from build123d import *

# Parameters (mm, degrees)
SKETCH_1_W          = 2.5
SKETCH_1_H          = 103
SKETCH_1_W_2        = 2
SKETCH_1_H_2        = 95
EXTRUDE_1_DEPTH     = 99.5
CUT_EXTRUDE_2_DEPTH = 4.5
CUT_EXTRUDE_3_DEPTH = 58.5
CUT_EXTRUDE_4_DEPTH = 4.5
SKETCH_6_W          = 1.6
SKETCH_6_H          = 17
CUT_EXTRUDE_5_DEPTH = 10
EXTRUDE_START       = -62
SKETCH_7_W          = 1
SKETCH_7_H          = 1
EXTRUDE_2_DEPTH     = 119.954657
EXTRUDE_START_2     = -58
SKETCH_8_W          = 0.5
SKETCH_8_H          = 0.5
EXTRUDE_3_DEPTH     = 119.954657


with BuildPart() as part:
    # 스케치1 → 보스-돌출1 (new body)
    with BuildSketch(Plane(origin=(0, 0, 0), x_dir=(1, 0, 0), z_dir=(0, 1, 0))):
        with Locations((1.25, -51.5)):
            Rectangle(SKETCH_1_W, SKETCH_1_H)
        with Locations((3.5, -51.5)):
            Rectangle(SKETCH_1_W_2, SKETCH_1_H_2)
    extrude(amount=EXTRUDE_1_DEPTH)

    # 스케치2 → 컷-돌출2 (cut)
    with BuildSketch(Plane(origin=(4.5, 0, 0), x_dir=(0, 0, -1), z_dir=(1, 0, 0))):
        with BuildLine():
            Line((-62, 10), (-62, 0))
            Line((-62, 0), (-41, 0))
            Line((-41, 0), (-41, 10))
            ThreePointArc((-41, 10), (-51.5, 20.5), (-62, 10))
        make_face()
    extrude(amount=-CUT_EXTRUDE_2_DEPTH, mode=Mode.SUBTRACT)

    # 스케치3 → 컷-돌출3 (cut)
    with BuildSketch(Plane(origin=(0, 99.5, 0), x_dir=(1, 0, 0), z_dir=(0, 1, 0))):
        Polygon((2.5, -4), (2.5, 0), (0, 0), (0, -103), (2.5, -103), (2.5, -99), (4.5, -99), (4.5, -4), align=None)
    extrude(amount=-CUT_EXTRUDE_3_DEPTH, mode=Mode.SUBTRACT)

    # 스케치4 → 컷-돌출4 (cut)
    with BuildSketch(Plane(origin=(0, 41, 0), x_dir=(1, 0, 0), z_dir=(0, 1, 0))):
        Polygon((4.5, -4), (2.5, -4), (2.5, 0), (0, 0), (0, -103), (2.5, -103), (2.5, -99), (4.5, -99), align=None)
    extrude(amount=-CUT_EXTRUDE_4_DEPTH, mode=Mode.SUBTRACT)

    # 스케치6 → 컷-돌출5 (cut)
    with BuildSketch(Plane.XZ):
        with Locations((0.8, 74)):
            Rectangle(SKETCH_6_W, SKETCH_6_H)
    extrude(amount=-CUT_EXTRUDE_5_DEPTH, mode=Mode.SUBTRACT)

    # 스케치7 → 보스-돌출2 (add)
    with BuildSketch(Plane(origin=(0, 0, 0), x_dir=(-1, 0, 0), z_dir=(0, 0, -1)).offset(EXTRUDE_START)):
        with Locations((-1.25, 1.524584525)):
            Rectangle(SKETCH_7_W, SKETCH_7_H)
        with Locations((-1.25, 11.524584525)):
            Rectangle(SKETCH_7_W, SKETCH_7_H)
        with Locations((-1.25, 21.524584525)):
            Rectangle(SKETCH_7_W, SKETCH_7_H)
        with Locations((-1.25, 31.524584525)):
            Rectangle(SKETCH_7_W, SKETCH_7_H)
    extrude(amount=EXTRUDE_2_DEPTH)

    # 스케치8 → 보스-돌출3 (add)
    with BuildSketch(Plane(origin=(0, 0, 4), x_dir=(-1, 0, 0), z_dir=(0, 0, -1)).offset(EXTRUDE_START_2)):
        with Locations((-3.5, 3.368615417)):
            Rectangle(SKETCH_8_W, SKETCH_8_H)
        with Locations((-3.5, 13.368615417)):
            Rectangle(SKETCH_8_W, SKETCH_8_H)
        with Locations((-3.5, 23.368615417)):
            Rectangle(SKETCH_8_W, SKETCH_8_H)
        with Locations((-3.5, 33.368615417)):
            Rectangle(SKETCH_8_W, SKETCH_8_H)
    extrude(amount=EXTRUDE_3_DEPTH)


solid = part.part
Geometry: final body of the model. Coordinates: model frame, mm. A direction names the side the tool comes from. Give positions to 0.01 mm unless a question says otherwise; leave off trailing zeros. Write each loop counter-clockwise with the first axis right and the second up, starting at its lowest first coordinate (ties: lowest second). Pieces come first, ordered by that corner, then holes. Notation, with made-up numbers: M -21,49 L 14,49 A22 cw 14,86 Z; hole C -35,61 d7. An arc over 180 degrees is marked long. Answer in a Markdown table with one row per item. Add a question column.
(1) First-contact query: pin 1 (1.1 mm diameter, centred on y = 21.5, z = -18, fed in from +X); pin 2 (0.5 mm diameter, centred on x = 1, z = -30.5, fed in from +Y); pin 3 (0.5 mm diameter, centred on x = 0.5, z = 70, fed in from -Y); pin 4 (3 mm diameter, centred on y = 17, z = -21, fed in from -X). Flat tips, straight axial feed; report the tip coordinate or a pass-through.
(2) Ray query, line 1 (Y direction, x = 3.65, z = -18); line 2 (Y direction, x = 1.4, z = -36); line 3 (Z direction, x = 1.1, y = 10.5). Return the intervals inside material, ascending.
(3) Section A-A on z = 51.5. Return loops of the section in (x, y).
(4) Section C-C on y = 25.5. Return loops of the section in (x, z), and give its area (4 significant figures).
(5) Mould query, pull axis Z, two halves, no side actions, for faces 4 (the flat face through (1, 18, 103)), 5 (the flat face through (2, 0, 82)), 6 (the cylindrical face through (2.3, 20.5, 51.3)). Classes: +Z half, -Z half, draft (parallel to the pull), parting line (faces both ways), or undercut.
(6) Section B-B on z = -22. State how many separate pieces and enclosed holes the cut face has, and give its area (3 significant figures).
(7) Reachability of faces 1 (the flat face through (1.6, 5, 74)), 2 (the flat face through (2.5, 18, 101)), 3 (the flat face through (2, 0, 20)) from +Z, -Z, +X, -X, +Y, -Y: full face, straight path, thin tool, end or side. Return the list, or none.
Result set:
| question | item | result |
|---|---|---|
| 1 | pin 1 | stops at x = 1.75 |
| 1 | pin 2 | stops at y = 32.02 |
| 1 | pin 3 | stops at y = 10 |
| 1 | pin 4 | passes through |
| 2 | line 1 | y = 3.12 to 3.62, 13.12 to 13.62, 23.12 to 23.62, 33.12 to 33.62 |
| 2 | line 2 | y = 1.02 to 2.02, 11.02 to 12.02, 21.02 to 22.02, 31.02 to 32.02 |
| 2 | line 3 | z = 0 to 41.01, 61.99 to 103 |
| 3 | outline | M 0,20.5 L 4.5,20.5 L 4.5,36.5 L 0,36.5 Z; M 0.75,1.02 L 1.75,1.02 L 1.75,2.02 L 0.75,2.02 Z; M 0.75,11.02 L 1.75,11.02 L 1.75,12.02 L 0.75,12.02 Z; M 3.25,3.12 L 3.75,3.12 L 3.75,3.62 L 3.25,3.62 Z; M 3.25,13.12 L 3.75,13.12 L 3.75,13.62 L 3.25,13.62 Z |
| 4 | outline | M 0,0 L 2.5,0 L 2.5,4 L 4.5,4 L 4.5,99 L 2.5,99 L 2.5,103 L 0,103 Z |
| 4 | area | 447.5 mm^2 |
| 5 | face 4 | +Z half |
| 5 | face 5 | draft |
| 5 | face 6 | undercut |
| 6 | separate pieces | 8 |
| 6 | enclosed holes | 0 |
| 6 | area | 5.00 mm^2 |
| 7 | face 1 | -X, -Y |
| 7 | face 2 | +Z, +X, +Y, -Y |
| 7 | face 3 | +Z, -Z, +X, -X, -Y |
